from build123d import *

# Parameters (mm, degrees)
SKETCH1_W                    = 45
SKETCH1_H                    = 5
SKETCH1_R                    = 1
BOSS_EXTRUDE1_DEPTH          = 2
SKETCH2_W                    = 1.9
SKETCH2_H                    = 1.65
BOSS_EXTRUDE2_DEPTH          = 5
CHAMFER1_SIZE                = 1
CHAMFER1_SIZE_2              = 0.577350269
LPATTERN1_COUNT              = 10
LPATTERN1_PITCH              = 3.8
CHAMFER1_OF_LPATTERN1_SIZE   = 1
CHAMFER1_OF_LPATTERN1_SIZE_2 = 0.577350269


with BuildPart() as part:
    # Sketch1 → Boss-Extrude1 (new body)
    with BuildSketch(Plane(origin=(0, 0, 0), x_dir=(1, 0, 0), z_dir=(0, 1, 0))):
        with Locations((22.5, -2.5)):
            Rectangle(SKETCH1_W, SKETCH1_H)
        with Locations(Location((2.5, -2.5, 0), (0, 0, 270))):
            Circle(SKETCH1_R, mode=Mode.SUBTRACT)
        with Locations(Location((42.5, -2.5, 0), (0, 0, 270))):
            Circle(SKETCH1_R, mode=Mode.SUBTRACT)
    extrude(amount=BOSS_EXTRUDE1_DEPTH)

    # Sketch2 → Boss-Extrude2 (add)
    with BuildSketch(Plane.XY.offset(5)):
        with Locations((5.95, 2.825)):
            Rectangle(SKETCH2_W, SKETCH2_H)
    boss_extrude2 = extrude(amount=-BOSS_EXTRUDE2_DEPTH)

    # Chamfer1
    # the kernel refuses this chamfer: 1, 0.577350269 mm, written as the material it takes off along each edge
    with BuildSketch(Plane(origin=(2.412914245, 3.65, 0), x_dir=(0, -0.9998132206222079, -0.019326765612700737), z_dir=(1, 0, 0))) as chamfer1_piece_1:
        Polygon((CHAMFER1_SIZE * 0.999813220622, -CHAMFER1_SIZE * 0.0193267656127), (-CHAMFER1_SIZE_2 * 0.019326765619, -CHAMFER1_SIZE_2 * 0.999813220951), (0, 0), align=None)
    extrude(amount=7.074171509, mode=Mode.SUBTRACT)
    with BuildSketch(Plane(origin=(2.412914245, 3.65, 5), x_dir=(0, -0.9998132206222079, 0.01932676561270115), z_dir=(1, 0, 0))) as chamfer1_piece_2:
        Polygon((CHAMFER1_SIZE * 0.999813220622, CHAMFER1_SIZE * 0.0193267656127), (-CHAMFER1_SIZE_2 * 0.019326765619, CHAMFER1_SIZE_2 * 0.999813220951), (0, 0), align=None)
    extrude(amount=7.074171509, mode=Mode.SUBTRACT)
    with BuildSketch(Plane(origin=(6.9, 3.65, 7.587085755), x_dir=(-0.9983227437537925, 0.0578938624026711, 0), z_dir=(0, 0, -1))) as chamfer1_piece_3:
        Polygon((CHAMFER1_SIZE_2 * 0.998322744082, -CHAMFER1_SIZE_2 * 0.0578938624217), (-CHAMFER1_SIZE * 0.0578938624027, -CHAMFER1_SIZE * 0.998322743754), (0, 0), align=None)
    extrude(amount=10.174171509, mode=Mode.SUBTRACT)
    with BuildSketch(Plane(origin=(5, 3.65, 7.587085755), x_dir=(-0.01932676561270115, -0.9998132206222079, 0), z_dir=(0, 0, -1))) as chamfer1_piece_4:
        Polygon((CHAMFER1_SIZE * 0.999813220622, -CHAMFER1_SIZE * 0.0193267656127), (-CHAMFER1_SIZE_2 * 0.019326765619, -CHAMFER1_SIZE_2 * 0.999813220951), (0, 0), align=None)
    extrude(amount=10.174171509, mode=Mode.SUBTRACT)

    # LPattern1: Boss-Extrude2 ×10
    with Locations(*[(i * LPATTERN1_PITCH, 0, 0) for i in range(1, LPATTERN1_COUNT)]):
        add(boss_extrude2)

    # Chamfer1 of LPattern1
    # the kernel refuses this chamfer: 1, 0.577350269 mm, written as the material it takes off along each edge
    with BuildSketch(Plane(origin=(6.212914245, 3.65, 0), x_dir=(0, -0.9998132206222079, -0.019326765612700737), z_dir=(1, 0, 0)), Plane(origin=(10.012914245, 3.65, 0), x_dir=(0, -0.9998132206222079, -0.019326765612700737), z_dir=(1, 0, 0)), Plane(origin=(13.812914245, 3.65, 0), x_dir=(0, -0.9998132206222079, -0.019326765612700737), z_dir=(1, 0, 0)), Plane(origin=(17.612914245, 3.65, 0), x_dir=(0, -0.9998132206222079, -0.019326765612700737), z_dir=(1, 0, 0)), Plane(origin=(21.412914245, 3.65, 0), x_dir=(0, -0.9998132206222079, -0.019326765612700737), z_dir=(1, 0, 0)), Plane(origin=(25.212914245, 3.65, 0), x_dir=(0, -0.9998132206222079, -0.019326765612700737), z_dir=(1, 0, 0)), Plane(origin=(29.012914245, 3.65, 0), x_dir=(0, -0.9998132206222079, -0.019326765612700737), z_dir=(1, 0, 0)), Plane(origin=(32.812914245, 3.65, 0), x_dir=(0, -0.9998132206222079, -0.019326765612700737), z_dir=(1, 0, 0)), Plane(origin=(36.612914245, 3.65, 0), x_dir=(0, -0.9998132206222079, -0.019326765612700737), z_dir=(1, 0, 0))) as chamfer1_of_lpattern1_piece_1:
        Polygon((CHAMFER1_OF_LPATTERN1_SIZE * 0.999813220622, -CHAMFER1_OF_LPATTERN1_SIZE * 0.0193267656127), (-CHAMFER1_OF_LPATTERN1_SIZE_2 * 0.019326765619, -CHAMFER1_OF_LPATTERN1_SIZE_2 * 0.999813220951), (0, 0), align=None)
    extrude(amount=7.074171509, mode=Mode.SUBTRACT)
    with BuildSketch(Plane(origin=(6.212914245, 3.65, 5), x_dir=(0, 0.0578938624026711, -0.9983227437537925), z_dir=(1, 0, 0)), Plane(origin=(10.012914245, 3.65, 5), x_dir=(0, 0.0578938624026711, -0.9983227437537925), z_dir=(1, 0, 0)), Plane(origin=(13.812914245, 3.65, 5), x_dir=(0, 0.0578938624026711, -0.9983227437537925), z_dir=(1, 0, 0)), Plane(origin=(17.612914245, 3.65, 5), x_dir=(0, 0.0578938624026711, -0.9983227437537925), z_dir=(1, 0, 0)), Plane(origin=(21.412914245, 3.65, 5), x_dir=(0, 0.0578938624026711, -0.9983227437537925), z_dir=(1, 0, 0)), Plane(origin=(25.212914245, 3.65, 5), x_dir=(0, 0.0578938624026711, -0.9983227437537925), z_dir=(1, 0, 0)), Plane(origin=(29.012914245, 3.65, 5), x_dir=(0, 0.0578938624026711, -0.9983227437537925), z_dir=(1, 0, 0)), Plane(origin=(32.812914245, 3.65, 5), x_dir=(0, 0.0578938624026711, -0.9983227437537925), z_dir=(1, 0, 0))) as chamfer1_of_lpattern1_piece_2:
        Polygon((CHAMFER1_OF_LPATTERN1_SIZE_2 * 0.998322744082, -CHAMFER1_OF_LPATTERN1_SIZE_2 * 0.0578938624217), (-CHAMFER1_OF_LPATTERN1_SIZE * 0.0578938624027, -CHAMFER1_OF_LPATTERN1_SIZE * 0.998322743754), (0, 0), align=None)
    extrude(amount=7.074171509, mode=Mode.SUBTRACT)
    with BuildSketch(Plane(origin=(10.7, 3.65, 7.587085755), x_dir=(-0.9983227437537925, 0.0578938624026711, 0), z_dir=(0, 0, -1)), Plane(origin=(14.5, 3.65, 7.587085755), x_dir=(-0.9983227437537925, 0.0578938624026711, 0), z_dir=(0, 0, -1)), Plane(origin=(18.3, 3.65, 7.587085755), x_dir=(-0.9983227437537925, 0.057893862402671276, 0), z_dir=(0, 0, -1)), Plane(origin=(22.1, 3.65, 7.587085755), x_dir=(-0.9983227437537925, 0.057893862402671276, 0), z_dir=(0, 0, -1)), Plane(origin=(25.9, 3.65, 7.587085755), x_dir=(-0.9983227437537925, 0.057893862402671276, 0), z_dir=(0, 0, -1)), Plane(origin=(29.7, 3.65, 7.587085755), x_dir=(-0.9983227437537925, 0.057893862402671276, 0), z_dir=(0, 0, -1)), Plane(origin=(33.5, 3.65, 7.587085755), x_dir=(-0.9983227437537927, 0.05789386240266986, 0), z_dir=(0, 0, -1)), Plane(origin=(37.3, 3.65, 7.587085755), x_dir=(-0.9983227437537927, 0.05789386240266986, 0), z_dir=(0, 0, -1)), Plane(origin=(41.1, 3.65, 7.587085755), x_dir=(-0.9983227437537927, 0.05789386240266986, 0), z_dir=(0, 0, -1))) as chamfer1_of_lpattern1_piece_3:
        Polygon((CHAMFER1_OF_LPATTERN1_SIZE_2 * 0.998322744082, -CHAMFER1_OF_LPATTERN1_SIZE_2 * 0.0578938624217), (-CHAMFER1_OF_LPATTERN1_SIZE * 0.0578938624027, -CHAMFER1_OF_LPATTERN1_SIZE * 0.998322743754), (0, 0), align=None)
    extrude(amount=10.174171509, mode=Mode.SUBTRACT)
    with BuildSketch(Plane(origin=(8.8, 3.65, 7.587085755), x_dir=(-0.01932676561270029, -0.9998132206222079, 0), z_dir=(0, 0, -1)), Plane(origin=(12.6, 3.65, 7.587085755), x_dir=(-0.01932676561270029, -0.9998132206222079, 0), z_dir=(0, 0, -1)), Plane(origin=(16.4, 3.65, 7.587085755), x_dir=(-0.01932676561270029, -0.9998132206222079, 0), z_dir=(0, 0, -1)), Plane(origin=(20.2, 3.65, 7.587085755), x_dir=(-0.01932676561270029, -0.9998132206222079, 0), z_dir=(0, 0, -1)), Plane(origin=(24, 3.65, 7.587085755), x_dir=(-0.01932676561270029, -0.9998132206222079, 0), z_dir=(0, 0, -1)), Plane(origin=(27.8, 3.65, 7.587085755), x_dir=(-0.01932676561270029, -0.9998132206222079, 0), z_dir=(0, 0, -1)), Plane(origin=(31.6, 3.65, 7.587085755), x_dir=(-0.0193267656127003, -0.9998132206222079, 0), z_dir=(0, 0, -1)), Plane(origin=(35.4, 3.65, 7.587085755), x_dir=(-0.01932676561270373, -0.9998132206222079, 0), z_dir=(0, 0, -1)), Plane(origin=(39.2, 3.65, 7.587085755), x_dir=(-0.01932676561270373, -0.9998132206222079, 0), z_dir=(0, 0, -1))) as chamfer1_of_lpattern1_piece_4:
        Polygon((CHAMFER1_OF_LPATTERN1_SIZE * 0.999813220622, -CHAMFER1_OF_LPATTERN1_SIZE * 0.0193267656127), (-CHAMFER1_OF_LPATTERN1_SIZE_2 * 0.019326765619, -CHAMFER1_OF_LPATTERN1_SIZE_2 * 0.999813220951), (0, 0), align=None)
    extrude(amount=10.174171509, mode=Mode.SUBTRACT)
    with BuildSketch(Plane(origin=(36.612914245, 3.65, 5), x_dir=(0, -0.9998132206222079, 0.01932676561270115), z_dir=(1, 0, 0))) as chamfer1_of_lpattern1_piece_5:
        Polygon((CHAMFER1_OF_LPATTERN1_SIZE * 0.999813220622, CHAMFER1_OF_LPATTERN1_SIZE * 0.0193267656127), (-CHAMFER1_OF_LPATTERN1_SIZE_2 * 0.019326765619, CHAMFER1_OF_LPATTERN1_SIZE_2 * 0.999813220951), (0, 0), align=None)
    extrude(amount=7.074171509, mode=Mode.SUBTRACT)


solid = part.part
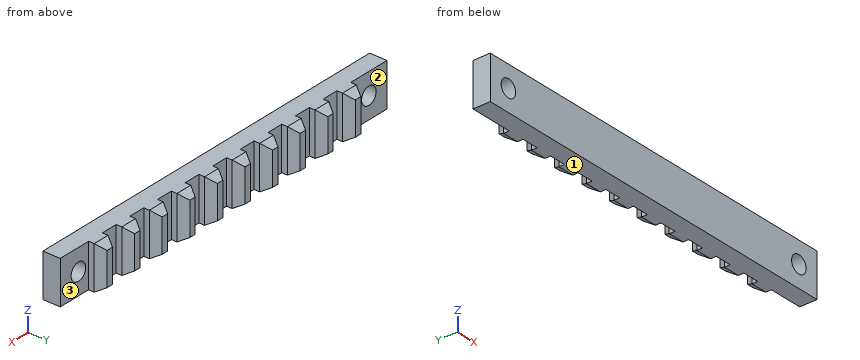
Check sheet for the modelled part. Datum: model origin and axes. Units: mm. Face numbers are marked on the shaded views. A direction names the side the tool comes from. Give positions to 0.01 mm unless a question says otherwise; leave off trailing zeros. Order: outer loops, then holes, each group sorted by start corner. A loop starts at its lowest first (then second) coordinate and runs counter-clockwise, first axis right, second up. Notation, with made-up numbers: M 9.25,17.25 L 56.25,17.25 A9 ccw 56.25,32.25 Z; hole C -11.75,-10.5 d11. An arc over 180 degrees is marked long. Answer as CSV lines item,"result". Start each with the question number.
Item 1: Cross-section at D-D on x = 19. Enter the section's corners in (y, z), plus the area to 3 significant figures.
Item 2: Cross-section at B-B on y = 1.2. Enter the section's corners in (x, z).
Item 3: Thickness scan on line 1 (X direction, y = 0.75, z = 2.5); line 2 (X direction, y = 0.85, z = 3.25); line 3 (Y direction, x = 19, z = 2.15). Record the ranges inside material, lowest first. Write a range as [from, to].
Item 4: Gauge pin test, flat ends, axial feed: P1, Ø2, axis at x = 38, z = 1.5, coming from the +Y side; P2, Ø0.5, axis at y = 2.5, z = 3, coming from the -X side; P3, Ø2, axis at x = 8, z = 2.5, coming from the +Y side. Record the tip position at first contact, or that the pin passes through.
Item 5: Tool access check on the marked faces 1, 2 and 3. Record the directions out of +Z, -Z, +X, -X, +Y, -Y that give a thin tool (end or side, any length) a straight path to the whole face; none if there is none.
Item 6: Cross-section at C-C on z = 3.1. State how many separate pieces and enclosed holes the cut face has, plus the area to 3 significant figures.
Item 7: Cross-section at A-A on x = 42.5. Enter the section's corners in (y, z).
Established:
1,outline,"M 0,0 L 2,0 L 2,5 L 0,5 Z"
1,area,"10.0 mm^2"
2,outline,"M 0,0 L 45,0 L 45,5 L 0,5 Z; hole C 2.5,2.5 d2; hole C 42.5,2.5 d2"
3,line 1,"x = [0, 1.5], [3.5, 41.5], [43.5, 45]"
3,line 2,"x = [0, 1.84], [3.16, 41.84], [43.16, 45]"
3,line 3,"y = [0, 2]"
4,P1,"stops at y = 3.17"
4,P2,"stops at x = 5"
4,P3,"stops at y = 3"
5,face 1,"-Z, +X, -X, +Y, -Y"
5,face 2,"+Z, -Z, -X, +Y"
5,face 3,"+Z, -Z, +X, +Y"
6,separate pieces,"3"
6,enclosed holes,"0"
6,area,"109 mm^2"
7,outline,"M 0,0 L 2,0 L 2,1.5 L 0,1.5 Z; M 0,3.5 L 2,3.5 L 2,5 L 0,5 Z"
